Build history of the part. All positions in model axes, mm. A direction names the side the tool comes from. Coordinates: 2 decimals unless noted, no trailing zeros. Order: outer loops, then holes, each group sorted by start corner. A loop starts at its lowest first (then second) coordinate and runs counter-clockwise, first axis right, second up. Notation, with made-up numbers: (62, 63) - (108, 63) arc R20 cw to (108, 67) - close; hole circle Ø3 at (-4.75, -26). An arc over 180 degrees is marked (long way). Write each question's results on one line, items separated by ' | '.
from build123d import *

# Parameters (mm, degrees)
SKETCH1_W           = 42
SKETCH1_H           = 14
BOSS_EXTRUDE1_DEPTH = 10
SHELL1_T            = -1.7
SKETCH2_W           = 1.7
SKETCH2_H           = 14
BOSS_EXTRUDE2_DEPTH = 5
SKETCH3_R           = 0.5
CUT_EXTRUDE1_DEPTH  = 13.3
CHAMFER1_SIZE       = 1
CHAMFER2_SIZE       = 1


with BuildPart() as part:
    # Sketch1 → Boss-Extrude1 (new body)
    with BuildSketch(Plane(origin=(0, 0, 0), x_dir=(1, 0, 0), z_dir=(0, 1, 0))):
        with Locations((19, 5)):
            Rectangle(SKETCH1_W, SKETCH1_H)
    extrude(amount=BOSS_EXTRUDE1_DEPTH)

    # Shell1
    shell1_openings = [part.faces().sort_by_distance(p)[0] for p in [
        (19, 10, -5),
    ]]
    offset(amount=SHELL1_T, openings=shell1_openings, kind=Kind.INTERSECTION)

    # Sketch2 → Boss-Extrude2 (add)
    with BuildSketch(Plane(origin=(0, 10, 0), x_dir=(1, 0, 0), z_dir=(0, 1, 0))):
        with Locations((-1.15, 5)):
            Rectangle(SKETCH2_W, SKETCH2_H)
        with Locations((39.15, 5)):
            Rectangle(SKETCH2_W, SKETCH2_H)
    extrude(amount=BOSS_EXTRUDE2_DEPTH)

    # Sketch3 → Cut-Extrude1 (cut)
    with BuildSketch(Plane(origin=(0, 15, 0), x_dir=(1, 0, 0), z_dir=(0, 1, 0))):
        with Locations((-0.3, 5)):
            Circle(SKETCH3_R)
        with Locations((38.3, 5)):
            Circle(SKETCH3_R)
    extrude(amount=-CUT_EXTRUDE1_DEPTH, mode=Mode.SUBTRACT)

    # Chamfer1
    chamfer1_edges = [part.edges().sort_by_distance(p)[0] for p in [
        (-0.3, 10, -11.15),
        (-0.3, 10, 1.15),
        (38.3, 10, -11.15),
        (38.3, 10, 1.15),
    ]]
    chamfer(chamfer1_edges, length=CHAMFER1_SIZE)

    # Chamfer2
    chamfer2_edges = [part.edges().sort_by_distance(p)[0] for p in [
        (19, 0, -12),
        (40, 0, -5),
        (19, 0, 2),
        (-2, 0, -5),
    ]]
    chamfer(chamfer2_edges, length=CHAMFER2_SIZE)


solid = part.part
1. Drop a flat-ended pin along its axis: pin 1 Ø1.9 at (x, z) = (22.5, -11.5) entering from +Y. Give the stop position or say it passes through.
Solved:
pin 1: stops at y = 10
2. Tool access for faces 4 (the face through (-0.3, 8, -2)), 5 (the face through (37.8, 10.5, 1.2)), 6 (the face through (39.5, 0.5, -4.9)): list every direction of +Z, -Z, +X, -X, +Y, -Y with a clear straight run to the whole face (end or side of a thin tool).
Solved:
face 4: +Y | face 5: +Z, -Z, +Y | face 6: +Z, -Z, +X, -Y
3. Probe line 1 (X direction, y = 7.75, z = -2); line 2 (Z direction, x = 20, y = 6); line 3 (X direction, y = 4.75, z = -5). List the from-to ranges inside material, lowest first.
Solved:
line 1: x = -2 to -0.3, 38.3 to 40 | line 2: z = -12 to -10.3, 0.3 to 2 | line 3: x = -2 to -0.8, 38.8 to 40
4. Band-saw the part on A-A on y = 12.75. Give the cut face in (x, z), then the cut area to 3 significant figures.
Solved:
outline: (-2, -12) - (-0.3, -12) - (-0.3, -5.5) arc R0.5 cw to (-0.3, -4.5) - (-0.3, 2) - (-2, 2) - close; (38.3, -12) - (40, -12) - (40, 2) - (38.3, 2) - (38.3, -4.5) arc R0.5 cw to (38.3, -5.5) - close | area: 46.8 mm2
5. Band-saw the part on C-C on z = -3.75. Give the cut face in (x, y), then the cut area to 3 significant figures.
Solved:
outline: (-2, 1) - (-1, 0) - (39, 0) - (40, 1) - (40, 15) - (38.3, 15) - (38.3, 1.7) - (-0.3, 1.7) - (-0.3, 15) - (-2, 15) - close | area: 116 mm2
6. Two-plate mould, pull along Z, no slides. Class faces 1 (the face through (19, 5, 2)), 2 (the face through (-0.8, 8.4, -5)), 3 (the face through (19, 10, 1)): +Z half, -Z half, draft (parallel to the pull), parting line (faces both ways), or undercut.
Solved:
face 1: +Z half | face 2: undercut | face 3: draft
7. Band-saw the part on B-B on x = 30.5. Give the cut face in (y, z).
Solved:
outline: (0, -11) - (1, -12) - (10, -12) - (10, -10.3) - (1.7, -10.3) - (1.7, 0.3) - (10, 0.3) - (10, 2) - (1, 2) - (0, 1) - close
